Design review of the part built by this model. Coordinates are the model's own, in mm. Face numbers are marked on the shaded views. Give positions to 0.01 mm unless a question says otherwise; leave off trailing zeros. Write each loop counter-clockwise with the first axis right and the second up, starting at its lowest first coordinate (ties: lowest second). Pieces come first, ordered by that corner, then holes.
```python
from build123d import *

# Parameters (mm, degrees)
PAD004_DEPTH            = 1.6
PAD005_DEPTH            = 1.6
LINEARPATTERN001_COUNT  = 2
LINEARPATTERN001_PITCH  = 8.4
FILLET004_R             = 1
FILLET005_R             = 1
FILLET006_R             = 1
FILLET007_R             = 1.5
PAD002_DEPTH            = 1.6
PAD003_DEPTH            = 1.6
LINEARPATTERN_COUNT     = 2
LINEARPATTERN_PITCH     = 8.4
FILLET_R                = 1
FILLET001_R             = 1
FILLET002_R             = 1
FILLET003_R             = 1.5
PAD008_DEPTH            = 1.6
PAD009_DEPTH            = 1.6
LINEARPATTERN003_COUNT  = 2
LINEARPATTERN003_PITCH  = 8.4
FILLET012_R             = 1
FILLET013_R             = 1
FILLET014_R             = 1
FILLET015_R             = 1.5
BODY004_PLACEMENT_ANGLE = 180
PAD006_DEPTH            = 1.6
PAD007_DEPTH            = 1.6
LINEARPATTERN002_COUNT  = 2
LINEARPATTERN002_PITCH  = 8.4
FILLET008_R             = 1
FILLET009_R             = 1
FILLET010_R             = 1
FILLET011_R             = 1.5
BODY003_PLACEMENT_ANGLE = 180
SKETCH_W                = 57
SKETCH_H                = 62
PAD_DEPTH               = 18
SKETCH001_W             = 54.6
SKETCH001_H             = 59.6
POCKET_DEPTH            = 16.8
SKETCH002_W             = 45
SKETCH002_H             = 3.5
POCKET001_DEPTH         = 57.001
SKETCH003_R             = 2.5
SKETCH003_R_2           = 0.9
PAD001_DEPTH            = 2.5
POCKET002_DEPTH         = 5


with BuildPart() as tab2:
    # Sketch006 → Pad004 (new body)
    with BuildSketch(Plane.XY):
        with BuildLine():
            Line((-4.5, 5), (4.5, 5))
            Line((4.5, 5), (4.5, 1.2))
            Line((0, 1.2), (4.5, 1.2))
            ThreePointArc((0, 1.2), (-1.2, 0), (0, -1.2))
            Line((4.5, -1.2), (0, -1.2))
            Line((4.5, -1.2), (4.5, -5))
            Line((4.5, -5), (-4.5, -5))
            Line((-4.5, -5), (-4.5, 5))
        make_face()
    extrude(amount=PAD004_DEPTH)

    # Sketch007 (on DatumPlane) → Pad005 (join)
    with BuildSketch(Plane.XZ.offset(5)):
        Polygon((-4.5, 0), (-4.5, -6), (-2.5, -6), (-2.5, -4.4), (0.5, 0), align=None)
    pad005 = extrude(amount=-PAD005_DEPTH)

    # LinearPattern001: Pad005 ×2
    with Locations(*[(0, i * LINEARPATTERN001_PITCH, 0) for i in range(1, LINEARPATTERN001_COUNT)]):
        add(pad005)

    # Fillet004
    fillet004_edges = [tab2.edges().sort_by_distance(p)[0] for p in [
        (-2.5, -4.2, -6),
        (-2.5, 4.2, -6),
    ]]
    fillet(fillet004_edges, radius=FILLET004_R)

    # Fillet005
    fillet005_edges = [tab2.edges().sort_by_distance(p)[0] for p in [
        (-2.5, -4.2, -4.4),
        (-2.5, 4.2, -4.4),
    ]]
    fillet(fillet005_edges, radius=FILLET005_R)

    # Fillet006
    fillet006_edges = [tab2.edges().sort_by_distance(p)[0] for p in [
        (4.5, -5, 0.8),
        (4.5, 5, 0.8),
    ]]
    fillet(fillet006_edges, radius=FILLET006_R)

    # Fillet007
    fillet007_edges = [tab2.edges().sort_by_distance(p)[0] for p in [
        (4.5, -1.2, 0.8),
        (4.5, 1.2, 0.8),
    ]]
    fillet(fillet007_edges, radius=FILLET007_R)


with BuildPart() as tab2_1:
    # Body002 placement: moved
    add(tab2.part.moved(Location((33, 22.5, 16.4))))


with BuildPart() as tab1:
    # Sketch004 → Pad002 (new body)
    with BuildSketch(Plane.XY):
        with BuildLine():
            Line((-4.5, 5), (4.5, 5))
            Line((4.5, 5), (4.5, 1.25))
            Line((0, 1.25), (4.5, 1.25))
            ThreePointArc((0, 1.25), (-1.25, 0), (0, -1.25))
            Line((4.5, -1.25), (0, -1.25))
            Line((4.5, -1.25), (4.5, -5))
            Line((4.5, -5), (-4.5, -5))
            Line((-4.5, -5), (-4.5, 5))
        make_face()
    extrude(amount=PAD002_DEPTH)

    # Sketch005 (on DatumPlane) → Pad003 (join)
    with BuildSketch(Plane.XZ.offset(5)):
        Polygon((-4.5, 0), (-4.5, -5.6), (-2.5, -5.6), (-2.5, -4), (0.5, 0), align=None)
    pad003 = extrude(amount=-PAD003_DEPTH)

    # LinearPattern: Pad003 ×2
    with Locations(*[(0, i * LINEARPATTERN_PITCH, 0) for i in range(1, LINEARPATTERN_COUNT)]):
        add(pad003)

    # Fillet
    fillet_edges = [tab1.edges().sort_by_distance(p)[0] for p in [
        (-2.5, -4.2, -5.6),
        (-2.5, 4.2, -5.6),
    ]]
    fillet(fillet_edges, radius=FILLET_R)

    # Fillet001
    fillet001_edges = [tab1.edges().sort_by_distance(p)[0] for p in [
        (-2.5, -4.2, -4),
        (-2.5, 4.2, -4),
    ]]
    fillet(fillet001_edges, radius=FILLET001_R)

    # Fillet002
    fillet002_edges = [tab1.edges().sort_by_distance(p)[0] for p in [
        (4.5, -5, 0.8),
        (4.5, 5, 0.8),
    ]]
    fillet(fillet002_edges, radius=FILLET002_R)

    # Fillet003
    fillet003_edges = [tab1.edges().sort_by_distance(p)[0] for p in [
        (4.5, -1.25, 0.8),
        (4.5, 1.25, 0.8),
    ]]
    fillet(fillet003_edges, radius=FILLET003_R)


with BuildPart() as tab1_1:
    # Body001 placement: moved
    add(tab1.part.moved(Location((33, -22.5, 16.4))))


with BuildPart() as tab4:
    # Sketch010 → Pad008 (new body)
    with BuildSketch(Plane.XY):
        with BuildLine():
            Line((-4.5, 5), (4.5, 5))
            Line((4.5, 5), (4.5, 1.25))
            Line((0, 1.25), (4.5, 1.25))
            ThreePointArc((0, 1.25), (-1.25, 0), (0, -1.25))
            Line((4.5, -1.25), (0, -1.25))
            Line((4.5, -1.25), (4.5, -5))
            Line((4.5, -5), (-4.5, -5))
            Line((-4.5, -5), (-4.5, 5))
        make_face()
    extrude(amount=PAD008_DEPTH)

    # Sketch011 (on DatumPlane) → Pad009 (join)
    with BuildSketch(Plane.XZ.offset(5)):
        Polygon((-4.5, 0), (-4.5, -6), (-2.5, -6), (-2.5, -4.4), (0.5, 0), align=None)
    pad009 = extrude(amount=-PAD009_DEPTH)

    # LinearPattern003: Pad009 ×2
    with Locations(*[(0, i * LINEARPATTERN003_PITCH, 0) for i in range(1, LINEARPATTERN003_COUNT)]):
        add(pad009)

    # Fillet012
    fillet012_edges = [tab4.edges().sort_by_distance(p)[0] for p in [
        (-2.5, -4.2, -6),
        (-2.5, 4.2, -6),
    ]]
    fillet(fillet012_edges, radius=FILLET012_R)

    # Fillet013
    fillet013_edges = [tab4.edges().sort_by_distance(p)[0] for p in [
        (-2.5, -4.2, -4.4),
        (-2.5, 4.2, -4.4),
    ]]
    fillet(fillet013_edges, radius=FILLET013_R)

    # Fillet014
    fillet014_edges = [tab4.edges().sort_by_distance(p)[0] for p in [
        (4.5, -5, 0.8),
        (4.5, 5, 0.8),
    ]]
    fillet(fillet014_edges, radius=FILLET014_R)

    # Fillet015
    fillet015_edges = [tab4.edges().sort_by_distance(p)[0] for p in [
        (4.5, -1.25, 0.8),
        (4.5, 1.25, 0.8),
    ]]
    fillet(fillet015_edges, radius=FILLET015_R)


with BuildPart() as tab4_1:
    # Body004 placement: moved
    add(tab4.part.moved(Location((-33, -22.5, 16.4))).rotate(Axis((-33, -22.5, 16.4), (0, 0, 1)), BODY004_PLACEMENT_ANGLE))


with BuildPart() as tab3:
    # Sketch008 → Pad006 (new body)
    with BuildSketch(Plane.XY):
        with BuildLine():
            Line((-4.5, 5), (4.5, 5))
            Line((4.5, 5), (4.5, 1.25))
            Line((0, 1.25), (4.5, 1.25))
            ThreePointArc((0, 1.25), (-1.25, 0), (0, -1.25))
            Line((4.5, -1.25), (0, -1.25))
            Line((4.5, -1.25), (4.5, -5))
            Line((4.5, -5), (-4.5, -5))
            Line((-4.5, -5), (-4.5, 5))
        make_face()
    extrude(amount=PAD006_DEPTH)

    # Sketch009 (on DatumPlane) → Pad007 (join)
    with BuildSketch(Plane.XZ.offset(5)):
        Polygon((-4.5, 0), (-4.5, -6), (-2.5, -6), (-2.5, -4.4), (0.5, 0), align=None)
    pad007 = extrude(amount=-PAD007_DEPTH)

    # LinearPattern002: Pad007 ×2
    with Locations(*[(0, i * LINEARPATTERN002_PITCH, 0) for i in range(1, LINEARPATTERN002_COUNT)]):
        add(pad007)

    # Fillet008
    fillet008_edges = [tab3.edges().sort_by_distance(p)[0] for p in [
        (-2.5, -4.2, -6),
        (-2.5, 4.2, -6),
    ]]
    fillet(fillet008_edges, radius=FILLET008_R)

    # Fillet009
    fillet009_edges = [tab3.edges().sort_by_distance(p)[0] for p in [
        (-2.5, -4.2, -4.4),
        (-2.5, 4.2, -4.4),
    ]]
    fillet(fillet009_edges, radius=FILLET009_R)

    # Fillet010
    fillet010_edges = [tab3.edges().sort_by_distance(p)[0] for p in [
        (4.5, -5, 0.8),
        (4.5, 5, 0.8),
    ]]
    fillet(fillet010_edges, radius=FILLET010_R)

    # Fillet011
    fillet011_edges = [tab3.edges().sort_by_distance(p)[0] for p in [
        (4.5, -1.25, 0.8),
        (4.5, 1.25, 0.8),
    ]]
    fillet(fillet011_edges, radius=FILLET011_R)


with BuildPart() as tab3_1:
    # Body003 placement: moved
    add(tab3.part.moved(Location((-33, 22.5, 16.4))).rotate(Axis((-33, 22.5, 16.4), (0, 0, 1)), BODY003_PLACEMENT_ANGLE))


with BuildPart() as body:
    # Sketch → Pad (new body)
    with BuildSketch(Plane.XY):
        Rectangle(SKETCH_W, SKETCH_H)
    extrude(amount=PAD_DEPTH)

    # Sketch001 (on DatumPlane) → Pocket (cut)
    with BuildSketch(Plane.XY.offset(18)):
        Rectangle(SKETCH001_W, SKETCH001_H)
    extrude(amount=-POCKET_DEPTH, mode=Mode.SUBTRACT)

    # Sketch002 (on Face3 of Pocket) → Pocket001 (cut, through all)
    with BuildSketch(Plane.YZ.offset(28.5)):
        with Locations((-0.5, 6.25)):
            Rectangle(SKETCH002_W, SKETCH002_H)
    extrude(amount=-POCKET001_DEPTH, mode=Mode.SUBTRACT)

    # Sketch003 (on Face19 of Pocket001) → Pad001 (join)
    with BuildSketch(Plane.XY.offset(1.2)):
        with Locations((22, -26.5)):
            Circle(SKETCH003_R)
        with Locations((22, -26.5)):
            Circle(SKETCH003_R_2, mode=Mode.SUBTRACT)
        with Locations((-22, -26.5)):
            Circle(SKETCH003_R)
        with Locations((-22, -26.5)):
            Circle(SKETCH003_R_2, mode=Mode.SUBTRACT)
        with Locations((22, 17.5)):
            Circle(SKETCH003_R)
        with Locations((22, 17.5)):
            Circle(SKETCH003_R_2, mode=Mode.SUBTRACT)
        with Locations((-22, 17.5)):
            Circle(SKETCH003_R)
        with Locations((-22, 17.5)):
            Circle(SKETCH003_R_2, mode=Mode.SUBTRACT)
    extrude(amount=PAD001_DEPTH)

    # Boolean: union Tab2, Tab1, Tab4, Tab3
    add(tab2_1.part)
    add(tab1_1.part)
    add(tab4_1.part)
    add(tab3_1.part)

    # Sketch012 (on DatumPlane) → Pocket002 (cut)
    with BuildSketch(Plane.XZ.offset(32)):
        with BuildLine():
            Line((-9.022841, 16.5), (9.022841, 16.5))
            ThreePointArc((10, 15.28749), (9.801465, 16.127491), (9.022841, 16.5))
            Line((9.72, 14), (10, 15.28749))
            Line((12.5, 14), (9.72, 14))
            ThreePointArc((12.5, 8.5), (15.25, 11.25), (12.5, 14))
            Line((12.5, 8.5), (8.84, 8.5))
            Line((8.5, 6.803495), (8.84, 8.5))
            ThreePointArc((7.519497, 6), (8.153333, 6.226532), (8.5, 6.803495))
            Line((-7.519497, 6), (7.519497, 6))
            ThreePointArc((-8.5, 6.803495), (-8.153333, 6.226532), (-7.519497, 6))
            Line((-8.84, 8.5), (-8.5, 6.803495))
            Line((-12.5, 8.5), (-8.84, 8.5))
            ThreePointArc((-12.5, 14), (-15.25, 11.25), (-12.5, 8.5))
            Line((-12.5, 14), (-9.72, 14))
            Line((-10, 15.28749), (-9.72, 14))
            ThreePointArc((-9.022841, 16.5), (-9.801465, 16.127491), (-10, 15.28749))
        make_face()
    extrude(amount=-POCKET002_DEPTH, mode=Mode.SUBTRACT)


solid = body.part
```
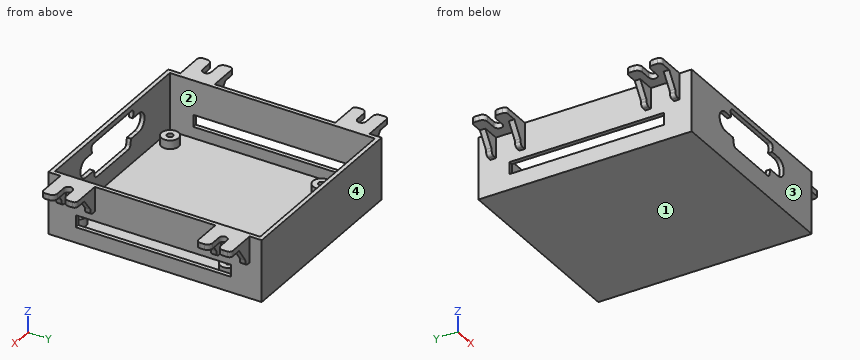
(1) Consider section A-A, the plane x = 2.5. Give the boundary of the cut face in (y, z), then the cut area to 3 significant figures.
Resolved:
outline: (-31, 0) - (31, 0) - (31, 18) - (29.8, 18) - (29.8, 1.2) - (-29.8, 1.2) - (-29.8, 6) - (-31, 6) - close; (-31, 16.5) - (-29.8, 16.5) - (-29.8, 18) - (-31, 18) - close
area: 102 mm2
(2) To check wall thickness, follow L1, parallel to Y at x = 22, z = 2.4; L2, parallel to X at y = -11, z = 17; L3, parallel to Y at x = -8.5, z = 2. State the ranges of each line that lie inside material, in increasing order.
Resolved:
L1: y = -31 to -29.8, -29 to -27.4, -25.6 to -24, 15 to 16.6, 18.4 to 20, 29.8 to 31
L2: x = -28.5 to -27.3, 27.3 to 28.5
L3: y = -31 to -29.8, 29.8 to 31
(3) Mouldability with a two-part tool opening along Y and no side actions: class the marked faces 1, 2, 3 and 4 as pulls with the +Y half, pulls with the -Y half, needs draft (parallel to the pull), parting line crosses it, or undercut.
Resolved:
face 1: needs draft
face 2: undercut
face 3: pulls with the -Y half
face 4: pulls with the +Y half
(4) Clearance check with flat-ended pins moving along their axes: P1, Ø1.3, axis at x = 34, z = 17, coming from the -Y side; P2, Ø0.5, axis at x = -22.5, y = 17.5, coming from the +Z side; P3, Ø8, axis at y = -24.5, z = 5, coming from the -X side. State where each tip first meets the part, or that it passes through.
Resolved:
P1: stops at y = -27.5
P2: stops at z = 1.2
P3: stops at x = -28.5
(5) Consider section D-D, the plane x = -22. Give the boundary of the cut face in (y, z).
Resolved:
outline: (-31, 0) - (31, 0) - (31, 18) - (29.8, 18) - (29.8, 1.2) - (20, 1.2) - (20, 3.7) - (18.4, 3.7) - (18.4, 1.2) - (16.6, 1.2) - (16.6, 3.7) - (15, 3.7) - (15, 1.2) - (-24, 1.2) - (-24, 3.7) - (-25.6, 3.7) - (-25.6, 1.2) - (-27.4, 1.2) - (-27.4, 3.7) - (-29, 3.7) - (-29, 1.2) - (-29.8, 1.2) - (-29.8, 18) - (-31, 18) - close
(6) Consider section C-C, the plane y = 5. Give the boundary of the cut face in (x, z), then the cut area to 3 significant figures.
Resolved:
outline: (-28.5, 0) - (28.5, 0) - (28.5, 4.5) - (27.3, 4.5) - (27.3, 1.2) - (-27.3, 1.2) - (-27.3, 4.5) - (-28.5, 4.5) - close; (-28.5, 8) - (-27.3, 8) - (-27.3, 18) - (-28.5, 18) - close; (27.3, 8) - (28.5, 8) - (28.5, 18) - (27.3, 18) - close
area: 100 mm2
(7) Consider section B-B, the plane z = 2. Give the number of separate pieces and of enclosed holes in the cut face, then the cut area to 3 significant figures.
Resolved:
separate pieces: 5
enclosed holes: 5
area: 348 mm2
